```python
from build123d import *

# Parameters (mm, degrees)
BOSS_EXTRUDE1_START = 21.4
SKETCH1_R           = 6.5
BOSS_EXTRUDE1_DEPTH = 2.1
BOSS_EXTRUDE2_START = 21.4
SKETCH2_W           = 20
SKETCH2_H           = 13
BOSS_EXTRUDE2_DEPTH = 2.1
CUT_EXTRUDE1_START  = 21.4
SKETCH3_R           = 3.55
CUT_EXTRUDE1_DEPTH  = 2.1
CUT_EXTRUDE2_START  = 21.4
CUT_EXTRUDE2_DEPTH  = 2.1


with BuildPart() as part:
    # Sketch1 → Boss-Extrude1 (new, symmetric)
    with BuildSketch(Plane(origin=(0, 0, 0), x_dir=(1, 0, 0), z_dir=(0, 1, 0)).offset(BOSS_EXTRUDE1_START)):
        with Locations(Location((0, 0, 0), (0, 0, 270))):
            Circle(SKETCH1_R)
    extrude(amount=BOSS_EXTRUDE1_DEPTH, both=True)

    # Sketch2 → Boss-Extrude2 (add, symmetric)
    with BuildSketch(Plane(origin=(0, 0, 0), x_dir=(1, 0, 0), z_dir=(0, 1, 0)).offset(BOSS_EXTRUDE2_START)):
        with Locations((10, 0)):
            Rectangle(SKETCH2_W, SKETCH2_H)
    extrude(amount=BOSS_EXTRUDE2_DEPTH, both=True)

    # Sketch3 → Cut-Extrude1 (cut, symmetric)
    with BuildSketch(Plane(origin=(0, 0, 0), x_dir=(1, 0, 0), z_dir=(0, 1, 0)).offset(CUT_EXTRUDE1_START)):
        with Locations(Location((0, 0, 0), (0, 0, 270))):
            Circle(SKETCH3_R)
    extrude(amount=CUT_EXTRUDE1_DEPTH, both=True, mode=Mode.SUBTRACT)

    # Sketch4 → Cut-Extrude2 (cut, symmetric)
    with BuildSketch(Plane(origin=(0, 0, 0), x_dir=(1, 0, 0), z_dir=(0, 1, 0)).offset(CUT_EXTRUDE2_START)):
        Polygon((0, -3.55), (12.7, -2.403281405), (12.7, 2.403281405), (0, 3.55), align=None)
    extrude(amount=CUT_EXTRUDE2_DEPTH, both=True, mode=Mode.SUBTRACT)


solid = part.part
```
Geometry: final body of the model. Coordinates: model frame, mm. A direction names the side the tool comes from. Round coordinates to 2 decimals unless told otherwise and drop trailing zeros. Write each loop counter-clockwise with the first axis right and the second up, starting at its lowest first coordinate (ties: lowest second). Pieces come first, ordered by that corner, then holes. Notation, with made-up numbers: (71.25, 19.25) -> (78.25, 19.25) arc R31 ccw to (78.25, 49.25) -> close; hole circle Ø8 at (74, -39). An arc over 180 degrees is marked (long way). Return JSON: item names as keys, results as strings.
Q1. First-contact query: pin 1 Ø1.3 at (y, z) = (22, 1) entering from -X. Flat tip, straight axial feed; report the tip coordinate or a pass-through.
From the geometry:
{"pin 1": "x = -6.49"}
Q2. Section D-D on x = -4. Return the cut outline in (y, z).
From the geometry:
{"outline": "(19.3, -5.12) -> (23.5, -5.12) -> (23.5, 5.12) -> (19.3, 5.12) -> close"}
Q3. Section A-A on z = 0. Return the cut outline in (x, y), and give its area (4 significant figures).
From the geometry:
{"outline": "(-6.5, 19.3) -> (-3.55, 19.3) -> (-3.55, 23.5) -> (-6.5, 23.5) -> close; (12.7, 19.3) -> (20, 19.3) -> (20, 23.5) -> (12.7, 23.5) -> close", "area": "43.05 mm2"}
Q4. Set-up query: faces 1 (the flat face through (6.75, 21.43, -2.94)), 2 (the flat face through (10, 19.3, 3)). Return all of +Z, -Z, +X, -X, +Y, -Y with unobstructed straight access to the full face (end or side cutting, diameter ignored); none if empty.
From the geometry:
{"face 1": "+Y, -Y", "face 2": "+Z, -Z, +X, -X, -Y"}
Q5. Ray query, line 1 (Z direction, x = 0, y = 20.45); line 2 (X direction, y = 22.4, z = 0); line 3 (X direction, y = 20.7, z = -2.25). Return the intervals inside material, ascending.
From the geometry:
{"line 1": "-6.5 to -3.55, 3.55 to 6.5", "line 2": "-6.5 to -3.55, 12.7 to 20", "line 3": "-6.1 to -2.75, 12.7 to 20"}
Q6. Mould query, pull axis X, two halves, no side actions, for faces 3 (the cylindrical face through (-3.55, 21.43, -0.09)), 4 (the cylindrical face through (-6.5, 21.4, -0.1)), 5 (the flat face through (20, 21, 0)). Classes: +X half, -X half, draft (parallel to the pull), parting line (faces both ways), or undercut.
From the geometry:
{"face 3": "undercut", "face 4": "-X half", "face 5": "+X half"}
Q7. Section C-C on y = 22.55. Return the cut outline in (x, z).
From the geometry:
{"outline": "(0, -6.5) -> (20, -6.5) -> (20, 6.5) -> (0, 6.5) arc R6.5 ccw to start; hole (0.64, -3.49) -> (12.7, -2.4) -> (12.7, 2.4) -> (0.64, 3.49) arc R3.55 ccw (long way) to start"}
Q8. Section B-B on x = 5.5. Return the cut outline in (y, z).
From the geometry:
{"outline": "(19.3, -6.5) -> (23.5, -6.5) -> (23.5, -3.05) -> (19.3, -3.05) -> close; (19.3, 3.05) -> (23.5, 3.05) -> (23.5, 6.5) -> (19.3, 6.5) -> close"}
